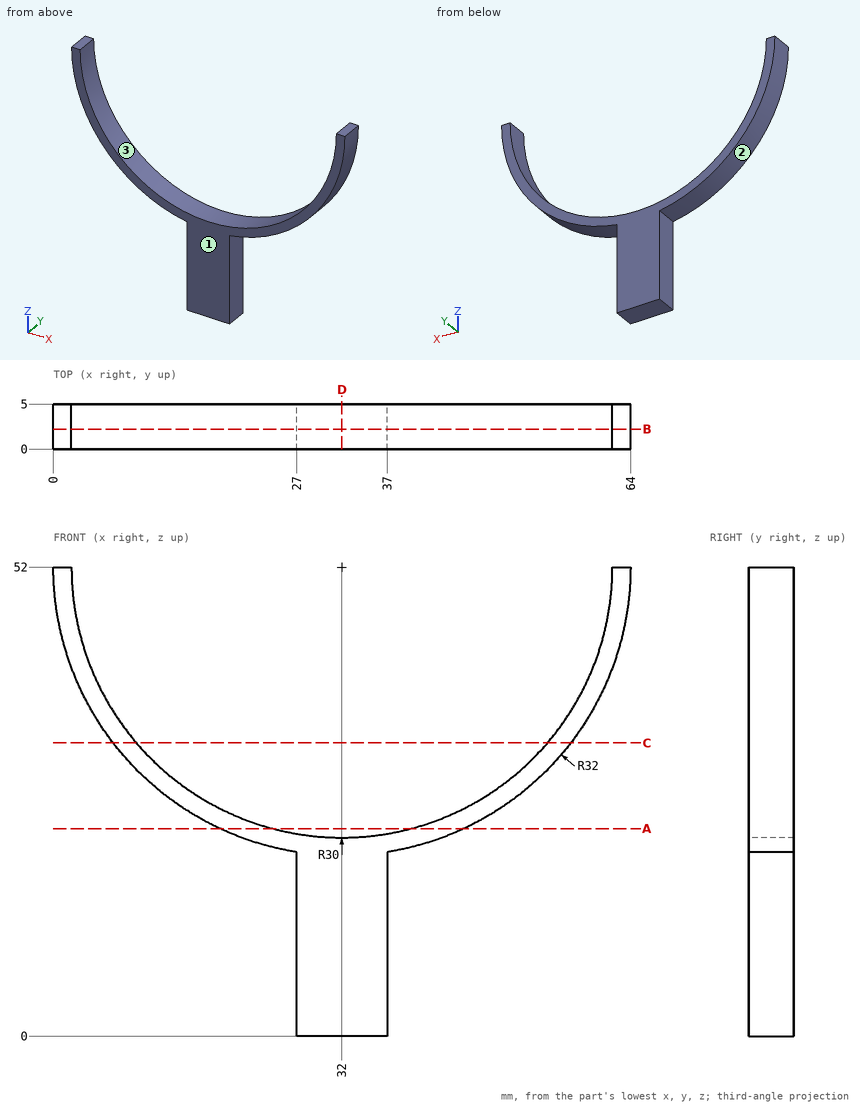
Study the drawing (mm; zero at the part's minimum x, y, z) and answer. Give positions to 0.01 mm unless a question says otherwise; leave off trailing zeros. Loops run counter-clockwise (first coordinate to the right, second up) from the corner with the lowest first, then second, coordinate; pieces in that order, holes last. Notation, with made-up numbers: (47, 69) - (84, 69) arc R28 cw to (84, 89) - close; hole circle Ø7 at (-31, 69.25). An arc over 180 degrees is marked (long way). Use CSV: the item, a comma, the result in double quotes. Start each with the question number.
(1) Find section A-A, the plane z = 23. Determine the outline of the cut face in (x, y).
(2) Find the intervals of material crossed by L1, parallel to X at y = 4.15, z = 45; L2, parallel to X at y = 3.2, z = 34.5; L3, parallel to X at y = 4.2, z = 6.5, in increasing order.
(3) Determine the mould class of the marked faces 1, 2 and 3 for opening direction X: released by +X, released by -X, zero draft, split by the parting line, or undercut.
(4) Find section C-C, the plane z = 32.5. Determine the outline of the cut face in (x, y), plus the area to 3 significant figures.
(5) Find section B-B, the plane y = 2.2. Determine the outline of the cut face in (x, z), plus the area to 3 significant figures.
(6) Each of these flat-tipped pins is pushed along its axis until it touches: pin 1 (3 mm diameter, centred on x = 27.5, z = 25, fed in from +Y); pin 2 (1.5 mm diameter, centred on y = 3, z = 46, fed in from -X). Where does it stop, or does it pass through?
(7) Find section D-D, the plane x = 32. Determine the outline of the cut face in (y, z), plus the area to 3 significant figures.
Results found:
1,outline,"(18.47, 0) - (24.32, 0) - (24.32, 5) - (18.47, 5) - close; (39.68, 0) - (45.53, 0) - (45.53, 5) - (39.68, 5) - close"
2,L1,"0.78 to 2.83, 61.17 to 63.22"
2,L2,"5.21 to 7.63, 56.37 to 58.79"
2,L3,"27 to 37"
3,face 1,"zero draft"
3,face 2,"released by -X"
3,face 3,"undercut"
4,outline,"(6.63, 0) - (9.2, 0) - (9.2, 5) - (6.63, 5) - close; (54.8, 0) - (57.37, 0) - (57.37, 5) - (54.8, 5) - close"
4,area,"25.7 mm^2"
5,outline,"(0, 52) arc R32 ccw to (27, 20.39) - (27, 0) - (37, 0) - (37, 20.39) arc R32 ccw to (64, 52) - (62, 52) arc R30 cw to (2, 52) - close"
5,area,"396 mm^2"
6,pin 1,"through"
6,pin 2,"x = 0.43"
7,outline,"(0, 0) - (5, 0) - (5, 22) - (0, 22) - close"
7,area,"110 mm^2"
